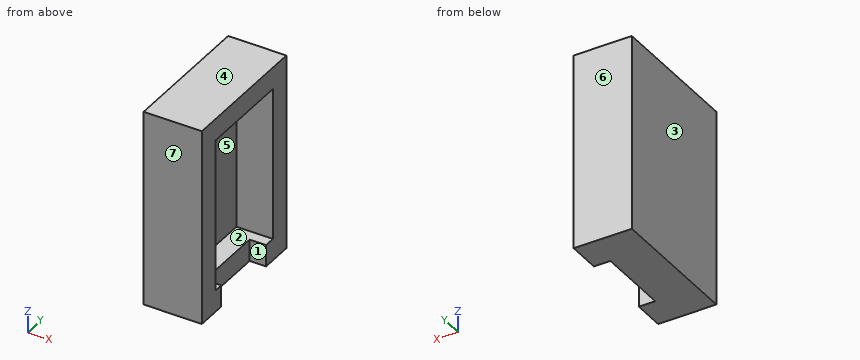
from build123d import *

# Parameters (mm, degrees)
SKETCH1_W           = 27
SKETCH1_H           = 19
BOSS_EXTRUDE1_DEPTH = 3
SKETCH2_W           = 27
SKETCH2_H           = 19
SKETCH2_W_2         = 21
SKETCH2_H_2         = 12.931843368
BOSS_EXTRUDE2_DEPTH = 5
SKETCH3_W           = 2.258281888
SKETCH3_H           = 10.091270109
CUT_EXTRUDE1_DEPTH  = 3


with BuildPart() as part:
    # Sketch1 → Boss-Extrude1 (new body)
    with BuildSketch(Plane(origin=(0, 0, 0), x_dir=(0, 0, -1), z_dir=(1, 0, 0))):
        Rectangle(SKETCH1_W, SKETCH1_H)
    extrude(amount=BOSS_EXTRUDE1_DEPTH)

    # Sketch2 → Boss-Extrude2 (add)
    with BuildSketch(Plane(origin=(3, 0, 0), x_dir=(0, 0, -1), z_dir=(1, 0, 0))):
        Rectangle(SKETCH2_W, SKETCH2_H)
        Rectangle(SKETCH2_W_2, SKETCH2_H_2, mode=Mode.SUBTRACT)
    extrude(amount=BOSS_EXTRUDE2_DEPTH)

    # Sketch3 → Cut-Extrude1 (cut)
    with BuildSketch(Plane(origin=(0, 0, -13.5), x_dir=(-1, 0, 0), z_dir=(0, 0, -1))):
        with Locations((-6.870859056, -0.117113387)):
            Rectangle(SKETCH3_W, SKETCH3_H)
    extrude(amount=-CUT_EXTRUDE1_DEPTH, mode=Mode.SUBTRACT)


solid = part.part
Source: CAD feature listing. Evaluate the final solid. Frame: model axes, mm. Face numbers are marked on the shaded views. A direction names the side the tool comes from. Coordinates: 2 decimals unless noted, no trailing zeros. Order: outer loops, then holes, each group sorted by start corner. A loop starts at its lowest first (then second) coordinate and runs counter-clockwise, first axis right, second up. Notation, with made-up numbers: M 49,18 L 97,18 A30 ccw 97,46 Z; hole C -6,-20 d1. An arc over 180 degrees is marked long. Write each question's results on one line, items separated by ' | '. Start each with the question number.
1. Section D-D, the plane x = 7.25. Return the cut outline in (y, z), then the cut area to 3 significant figures.
2. Section B-B, the plane y = 1. Return the cut outline in (x, z).
3. Section C-C, the plane z = -8.75. Return the cut outline in (x, y).
4. Draft query along Y for the marked faces 4, 5, 6 and 7. Return one class per face: +Y half, -Y half, draft (parallel to the pull), parting line (faces both ways), or undercut.
5. Pin query (flat end, axial travel): pin 1 (1 mm diameter, centred on y = 6.5, z = -1, fed in from -X); pin 2 (6.5 mm diameter, centred on y = 2, z = 2.5, fed in from +X); pin 3 (2.5 mm diameter, centred on y = 1, z = -11.5, fed in from +X). Return the tip coordinate at first contact, or that it passes through.
6. Section A-A, the plane x = 5. Return the cut outline in (y, z), then the cut area to 3 significant figures.
7. Reachability of the marked faces 1, 2 and 3 from +Z, -Z, +X, -X, +Y, -Y: full face, straight path, thin tool, end or side. Return the list, or none.
8. Material intervals for L1, parallel to Y at x = 4.25, z = 4.25; L2, parallel to Y at x = 6.75, z = -11.5; L3, parallel to Z at x = 5.25, y = 1.5, sorted ascending.
Solution:
1) outline: M -9.5,-13.5 L -5.16,-13.5 L -5.16,-10.5 L -6.47,-10.5 L -6.47,10.5 L 6.47,10.5 L 6.47,-10.5 L 4.93,-10.5 L 4.93,-13.5 L 9.5,-13.5 L 9.5,13.5 L -9.5,13.5 Z | area: 211 mm²
2) outline: M 0,-13.5 L 5.74,-13.5 L 5.74,-10.5 L 3,-10.5 L 3,10.5 L 8,10.5 L 8,13.5 L 0,13.5 Z
3) outline: M 0,-9.5 L 8,-9.5 L 8,-6.47 L 3,-6.47 L 3,6.47 L 8,6.47 L 8,9.5 L 0,9.5 Z
4) face 4: draft | face 5: undercut | face 6: +Y half | face 7: -Y half
5) pin 1: x = 0 | pin 2: x = 3 | pin 3: x = 5.74
6) outline: M -9.5,-13.5 L 9.5,-13.5 L 9.5,13.5 L -9.5,13.5 Z; hole M -6.47,-10.5 L 6.47,-10.5 L 6.47,10.5 L -6.47,10.5 Z | area: 241 mm²
7) face 1: -Z, +X | face 2: +X | face 3: +Z, -Z, -X, +Y, -Y
8) L1: -9.5 to -6.47, 6.47 to 9.5 | L2: -9.5 to -5.16, 4.93 to 9.5 | L3: -13.5 to -10.5, 10.5 to 13.5
